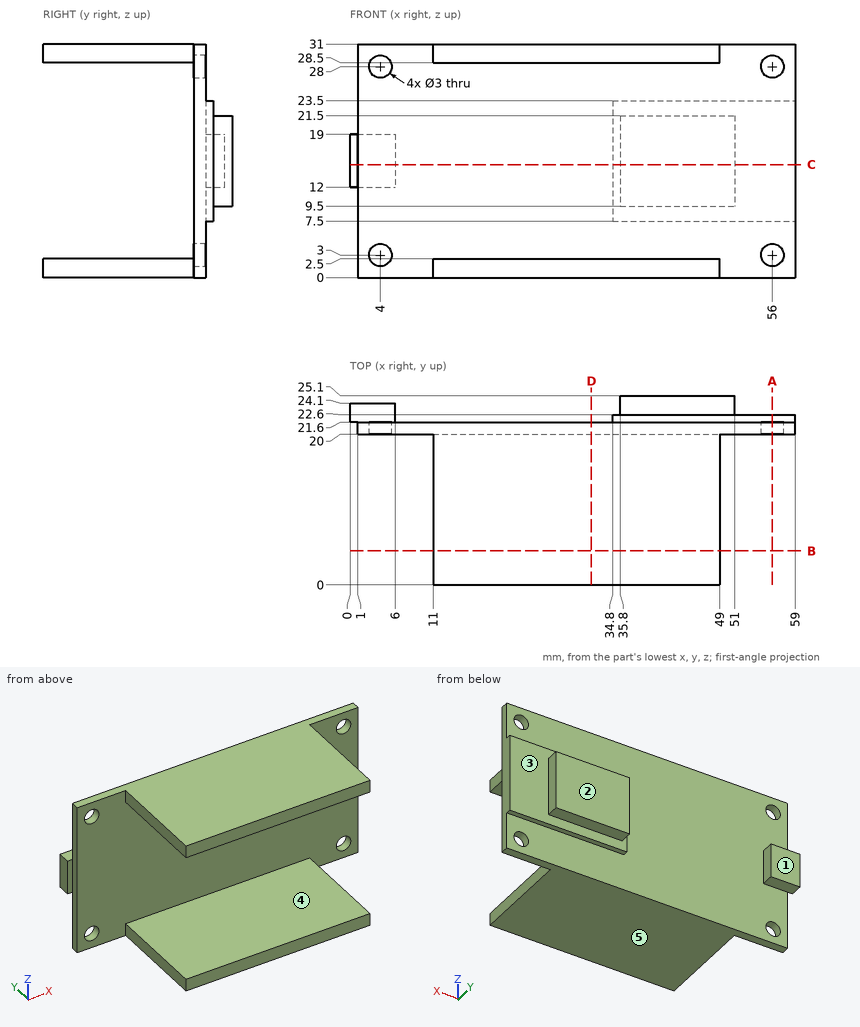
Geometry check sheet. Reference: drawing and pictorial views, mm from the part's lowest x, y, z. A direction names the side the tool comes from. Coordinates: 2 decimals unless noted, no trailing zeros. Order: outer loops, then holes, each group sorted by start corner. A loop starts at its lowest first (then second) coordinate and runs counter-clockwise, first axis right, second up. Notation, with made-up numbers: M 65,17 L 106,17 A4 cw 106,22 Z; hole C -30,3.5 d5. An arc over 180 degrees is marked long. Return JSON: item names as keys, results as strings.
1) Thickness scan on L1, parallel to X at y = 21.2, z = 3; L2, parallel to Z at x = 44.5, y = 12; L3, parallel to Y at x = 6.5, z = 17. Record the ranges inside material, lowest first. Write a range as [from, to].
Answer list:
{"L1": "[1, 2.5], [5.5, 54.5], [57.5, 59]", "L2": "[0, 2.5], [28.5, 31]", "L3": "[20, 21.6]"}
2) Cross-section at B-B, the plane y = 4.5. Record the boundary of the cut face in (x, z).
Answer list:
{"outline": "M 11,0 L 49,0 L 49,2.5 L 11,2.5 Z; M 11,28.5 L 49,28.5 L 49,31 L 11,31 Z"}
3) Release check for a two-part mould opening along Z. For the marked faces 3, 4 and 5 record: +Z half, -Z half, draft (parallel to the pull), parting line (faces both ways), or undercut.
Answer list:
{"face 3": "draft", "face 4": "undercut", "face 5": "-Z half"}
4) Cross-section at C-C, the plane z = 15. Record the boundary of the cut face in (x, y), and give its area (3 significant figures).
Answer list:
{"outline": "M 0,21.6 L 1,21.6 L 1,20 L 59,20 L 59,22.6 L 51,22.6 L 51,25.1 L 35.8,25.1 L 35.8,22.6 L 34.8,22.6 L 34.8,21.6 L 6,21.6 L 6,24.1 L 0,24.1 Z", "area": "170 mm2"}
5) Cross-section at A-A, the plane x = 56. Record the boundary of the cut face in (y, z).
Answer list:
{"outline": "M 20,0 L 21.6,0 L 21.6,1.5 L 20,1.5 Z; M 20,4.5 L 21.6,4.5 L 21.6,7.5 L 22.6,7.5 L 22.6,23.5 L 21.6,23.5 L 21.6,26.5 L 20,26.5 Z; M 20,29.5 L 21.6,29.5 L 21.6,31 L 20,31 Z"}
6) Access from +Z, -Z, +X, -X, +Y, -Y to the whole of each face (thin tool, end or side, straight path). Record for the marked faces 1 and 2.
Answer list:
{"face 1": "+Z, -Z, -X, +Y", "face 2": "+Z, -Z, +X, -X, +Y"}
7) Cross-section at D-D, the plane x = 32. Record the boundary of the cut face in (y, z).
Answer list:
{"outline": "M 0,0 L 21.6,0 L 21.6,31 L 0,31 L 0,28.5 L 20,28.5 L 20,2.5 L 0,2.5 Z"}
8) Gauge pin test, flat ends, axial feed: pin 1 (2 mm diameter, centred on x = 41, y = 24, fed in from +Z); pin 2 (2 mm diameter, centred on y = 9, z = 1.5, fed in from +X); pin 3 (3 mm diameter, centred on x = 2.5, z = 14, fed in from +Y). Record the tip position at first contact, or that the pin passes through.
Answer list:
{"pin 1": "z = 21.5", "pin 2": "x = 49", "pin 3": "y = 24.1"}
